```python
from build123d import *

# Parameters (mm, degrees)
F1_DEPTH  = 38.1
F2_W      = 66.04
F2_H      = 9.525
F3_DEPTH  = 15.24
F2_H_2    = 6.35
F4_DEPTH  = 30.48
F5_DEPTH  = 15.24
F6_W      = 19.05
F6_H      = 5.08
F7_DEPTH  = 3.175
F9_DEPTH  = 6.35
F11_DEPTH = 3.175
F13_DEPTH = 1.27


with BuildPart() as f1:
    # F0 (on Front) → F1 (new body, symmetric)
    with BuildSketch(Plane.XZ):
        Polygon((-0.8076530991, -1.0001709495), (0, 0), (-60.1146014221, 34.7071813133), (-60.7496014221, 33.6073290505), align=None)
    extrude(amount=F1_DEPTH, both=True)

    # F2 (on face) → F3 (join)
    with BuildSketch(Plane(origin=(0, 0, 0), x_dir=(0.8660254038, 0, -0.5), z_dir=(0.5, 0, 0.8660254038))):
        with Locations((-36.195, -14.2875)):
            Rectangle(F2_W, F2_H)
        with Locations((-36.195, 14.2875)):
            Rectangle(F2_W, F2_H)
    extrude(amount=F3_DEPTH)

    # F2 (on face) → F4 (join)
    with BuildSketch(Plane(origin=(0, 0, 0), x_dir=(0.8660254038, 0, -0.5), z_dir=(0.5, 0, 0.8660254038))):
        with Locations((-36.195, -22.225)):
            Rectangle(F2_W, F2_H_2)
        with Locations((-36.195, 22.225)):
            Rectangle(F2_W, F2_H_2)
    extrude(amount=F4_DEPTH)

    # F2 (on face) → F5 (join)
    with BuildSketch(Plane(origin=(0, 0, 0), x_dir=(0.8660254038, 0, -0.5), z_dir=(0.5, 0, 0.8660254038))):
        Polygon((0, 25.4), (-3.175, 25.4), (-3.175, 19.05), (-3.175, 9.525), (-3.175, -9.525), (-3.175, -19.05), (-3.175, -25.4), (0, -25.4), align=None)
    extrude(amount=F5_DEPTH)

    # F6 (on face) → F7 (cut)
    with BuildSketch(Plane(origin=(0, 0, 0), x_dir=(0, 1, 0), z_dir=(0.8660254038, 0, -0.5))):
        with Locations((0, 2.54)):
            Rectangle(F6_W, F6_H)
    extrude(amount=-F7_DEPTH, mode=Mode.SUBTRACT)

    # F8 (on face) → F9 (join)
    with BuildSketch(Plane.XZ.offset(38.1)):
        Polygon((-60.7496014221, -1.0001709495), (-0.8076530991, -1.0001709495), (-60.7496014221, 33.6073290505), align=None)
    extrude(amount=-F9_DEPTH)

    # F10 (on face) → F11 (join)
    with BuildSketch(Plane(origin=(0, 38.1, 0), x_dir=(-1, 0, 0), z_dir=(0, 1, 0))):
        Polygon((60.7496014221, 33.6073290505), (0.8076530991, -1.0001709495), (60.6936737895, -1.0001709495), align=None)
    extrude(amount=-F11_DEPTH)

    # F12 (on face) → F13 (join)
    with BuildSketch(Plane(origin=(0, 0, -1.0001709495), x_dir=(1, 0, 0), z_dir=(0, 0, -1))):
        Polygon((0, 49.53), (-60.7496014221, 49.53), (-60.7496014221, 38.1), (-0.8076530991, 38.1), (-0.8076530991, 31.75), (-60.7496014221, 31.75), (-60.7496014221, -49.53), (0, -49.53), (0, -9.525), (0, 9.525), align=None)
    extrude(amount=-F13_DEPTH)


solid = f1.part
```
Part model, mm, in its own coordinate system. A direction names the side the tool comes from. Round coordinates to 2 decimals unless told otherwise and drop trailing zeros. Write each loop counter-clockwise with the first axis right and the second up, starting at its lowest first coordinate (ties: lowest second). Pieces come first, ordered by that corner, then holes.
Item 1: Probe L1, parallel to Y at x = -3, z = 25; L2, parallel to Y at x = -6.5, z = 13 (3 decimals); L3, parallel to X at y = -0.5, z = 9. List the from-to ranges inside material, lowest first.
Results:
L1: y = -25.4 to -19.05, 19.05 to 25.4
L2: y = -25.4 to -9.525, 9.525 to 25.4
L3: x = -18.13 to -15.59, 1.53 to 5.2
Item 2: Cut at B-B, the plane x = 6. Give the cut face in (y, z).
Results:
outline: (-25.4, 10.39) - (25.4, 10.39) - (25.4, 14.13) - (-25.4, 14.13) - close; (-25.4, 16.74) - (-19.05, 16.74) - (-19.05, 31.73) - (-25.4, 31.73) - close; (19.05, 16.74) - (25.4, 16.74) - (25.4, 31.73) - (19.05, 31.73) - close
Item 3: Which spindle directions (+Z, -Z, +X, -X, +Y, -Y) get a long thin tool onto all of the face, cutting with end or side? Do faces 4 (the flat face through (8.627, -22.269, 21.292)), 5 (the flat face through (-44, 38.1, 10)), 6 (the flat face through (-38, -38.1, 14)). Say none if no direction does.
Results:
face 4: +X, +Y, -Y
face 5: +Z, +X, -X, +Y
face 6: +Z, +X, -X, -Y
Item 4: Cut at D-D, the plane z = 12. Give the cut face in (x, y) (3 decimals), plus the area to 3 significant figures.
Results:
outline: (-60.75, -38.1) - (-20.785, -38.1) - (-20.785, -25.4) - (6.928, -25.4) - (6.928, 25.4) - (-20.785, 25.4) - (-20.785, 38.1) - (-60.715, 38.1) - (-60.715, 34.925) - (-23.325, 34.925) - (-23.325, -31.75) - (-60.75, -31.75) - close; hole (-20.785, -9.525) - (3.262, -9.525) - (3.262, 9.525) - (-20.785, 9.525) - close
area: 1,500 mm2
Item 5: Drop flat-ended pins along their axis: pin 1 Ø1 at (y, z) = (4.5, 0) entering from +X; pin 2 Ø7 at (x, y) = (-38.5, -35) entering from +Z; pin 3 Ø4 at (y, z) = (-5.5, 19.5) entering from -X. Give the stop position or say it passes through.
Results:
pin 1: stops at x = 0
pin 2: stops at z = 24.25
pin 3: stops at x = -39.78
Item 6: Two-plate mould, pull along Z, no slides. Class faces 1 (the flat face through (-60.75, -33, 11)), 2 (the flat face through (-45, -31.75, 10)), 3 (the flat face through (2.29, 0.13, 10.32)): +Z half, -Z half, draft (parallel to the pull), parting line (faces both ways), or undercut.
Results:
face 1: draft
face 2: undercut
face 3: +Z half
Item 7: Cut at C-C, the plane y = -17. Give the cut face in (x, z), plus the area to 3 significant figures.
Results:
outline: (-60.75, -1) - (0, -1) - (0, 0) - (7.62, 13.2) - (-52.32, 47.81) - (-59.94, 34.61) - (-60.11, 34.71) - (-60.75, 33.61) - (-3.01, 0.27) - (-60.75, 0.27) - close
area: 1,220 mm2
Item 8: Cut at A-A, the plane y = 0.5. Give the cut face in (x, z), plus the area to 3 significant figures.
Results:
outline: (-60.75, -1) - (0, -1) - (0, 0.27) - (-0.47, 0.27) - (-60.11, 34.71) - (-60.75, 33.61) - (-3.01, 0.27) - (-60.75, 0.27) - close; (-0.21, 5.99) - (2.54, 4.4) - (7.62, 13.2) - (4.87, 14.79) - close
area: 195 mm2
